from build123d import *

# Parameters (mm, degrees)
SKETCH_1_R      = 1.6
SKETCH_1_R_2    = 2.4
EXTRUDE_1_DEPTH = 3.2
CHAMFER_1_SIZE  = 1.4


with BuildPart() as part:
    # 草图1 → 凸台-拉伸1 (new body)
    with BuildSketch(Plane.XY):
        with BuildLine():
            Line((-20, 20), (20, 20))
            ThreePointArc((20, 20), (40, 0), (20, -20))
            Line((20, -20), (-20, -20))
            ThreePointArc((-20, -20), (-40, 0), (-20, 20))
        make_face()
        with Locations((-19, -14)):
            Circle(SKETCH_1_R, mode=Mode.SUBTRACT)
        with Locations((19, -14)):
            Circle(SKETCH_1_R, mode=Mode.SUBTRACT)
        with Locations((19, 6)):
            Circle(SKETCH_1_R, mode=Mode.SUBTRACT)
        with Locations((-19, 6)):
            Circle(SKETCH_1_R, mode=Mode.SUBTRACT)
        with Locations((-10, 0)):
            Circle(SKETCH_1_R_2, mode=Mode.SUBTRACT)
        with Locations((10, 0)):
            Circle(SKETCH_1_R_2, mode=Mode.SUBTRACT)
    extrude(amount=EXTRUDE_1_DEPTH)

    # 倒角1
    chamfer_1_edges = [part.edges().sort_by_distance(p)[0] for p in [
        (-20.6, -14, 3.2),
        (17.4, -14, 3.2),
        (17.4, 6, 3.2),
        (-20.6, 6, 3.2),
    ]]
    chamfer(chamfer_1_edges, length=CHAMFER_1_SIZE)


solid = part.part
For this review, take the finished solid that the model builds, in its own axes (mm). Coordinates: 2 decimals unless noted, no trailing zeros. Loops run counter-clockwise (first coordinate to the right, second up) from the corner with the lowest first, then second, coordinate; pieces in that order, holes last. Notation, with made-up numbers: (30, 38) - (77, 38) arc R22 cw to (77, 63) - close; hole circle Ø3 at (-39, 60.25). An arc over 180 degrees is marked (long way). Use a Markdown table: item, result. Add a question column.
Item 1: We need section D-D (y = 12). Give the boundary of the cut face in (x, z), and give its area (3 significant figures).
Item 2: We need section A-A (y = 0). Give the boundary of the cut face in (x, z).
Item 3: For line 1 (Y direction, x = 19, z = 0.6); line 2 (Y direction, x = -16.5, z = 3); line 3 (Y direction, x = 10, z = 3), list the stretches that pass through material, from the lowest coordinate up.
Item 4: We need section C-C (x = 10). Give the boundary of the cut face in (y, z).
Item 5: Mouldability with a two-part tool opening along X and no side actions: class faces 1 (the face through (0, 20, 2)), 2 (the face through (-20.18, -12.92, 0.89)), 3 (the face through (-40, 0, 2)) as pulls with the +X half, pulls with the -X half, needs draft (parallel to the pull), parting line crosses it, or undercut.
Item 6: We need section B-B (x = -19). Give the boundary of the cut face in (y, z).
Item 7: Insertion check: pin 1 Ø4 at (x, y) = (10, 0) entering from +Z; pin 2 Ø4 at (x, y) = (-5.5, 7.5) entering from -Z; pin 3 Ø3.5 at (x, y) = (-19, 6) entering from +Z; pin 4 Ø1.5 at (y, z) = (3.5, 2) entering from +X. Each pin has a flat end and moves straight along its axis. Give the tip position at first contact, or say it passes through.
Results list:
| question | item | result |
|---|---|---|
| 1 | outline | (-36, 0) - (36, 0) - (36, 3.2) - (-36, 3.2) - close |
| 1 | area | 230 mm^2 |
| 2 | outline | (-40, 0) - (-12.4, 0) - (-12.4, 3.2) - (-40, 3.2) - close; (-7.6, 0) - (7.6, 0) - (7.6, 3.2) - (-7.6, 3.2) - close; (12.4, 0) - (40, 0) - (40, 3.2) - (12.4, 3.2) - close |
| 3 | line 1 | y = -20 to -15.6, -12.4 to 4.4, 7.6 to 20 |
| 3 | line 2 | y = -20 to -15.26, -12.74 to 4.74, 7.26 to 20 |
| 3 | line 3 | y = -20 to -2.4, 2.4 to 20 |
| 4 | outline | (-20, 0) - (-2.4, 0) - (-2.4, 3.2) - (-20, 3.2) - close; (2.4, 0) - (20, 0) - (20, 3.2) - (2.4, 3.2) - close |
| 5 | face 1 | needs draft |
| 5 | face 2 | undercut |
| 5 | face 3 | pulls with the -X half |
| 6 | outline | (-20, 0) - (-15.6, 0) - (-15.6, 1.8) - (-17, 3.2) - (-20, 3.2) - close; (-12.4, 0) - (4.4, 0) - (4.4, 1.8) - (3, 3.2) - (-11, 3.2) - (-12.4, 1.8) - close; (7.6, 0) - (20, 0) - (20, 3.2) - (9, 3.2) - (7.6, 1.8) - close |
| 7 | pin 1 | passes through |
| 7 | pin 2 | stops at z = 0 |
| 7 | pin 3 | stops at z = 1.95 |
| 7 | pin 4 | stops at x = 39.81 |
